from build123d import *

# Parameters (mm, degrees)
F0_R     = 39.5
F0_R_2   = 10.25
F1_DEPTH = 2
F2_R     = 11.25
F2_R_2   = 10.25
F3_DEPTH = 68
F4_R     = 12.5
F5_DEPTH = 1
F6_R     = 39.5
F6_R_2   = 10.25
F7_DEPTH = 2
F8_R     = 12.5
F9_DEPTH = 1


with BuildPart() as f1:
    # F0 (on Front) → F1 (new body)
    with BuildSketch(Plane.XZ):
        Circle(F0_R)
        Circle(F0_R_2, mode=Mode.SUBTRACT)
    extrude(amount=F1_DEPTH)

    # F2 (on face) → F3 (join)
    with BuildSketch(Plane.XZ.offset(2)):
        Circle(F2_R)
        Circle(F2_R_2, mode=Mode.SUBTRACT)
    extrude(amount=F3_DEPTH)

    # F4 (on face) → F5 (cut)
    with BuildSketch(Plane(origin=(0, 0, 0), x_dir=(-1, 0, 0), z_dir=(0, 1, 0))):
        Circle(F4_R)
    extrude(amount=-F5_DEPTH, mode=Mode.SUBTRACT)

    # F6 (on face) → F7 (join)
    with BuildSketch(Plane.XZ.offset(70)):
        Circle(F6_R)
        Circle(F6_R_2, mode=Mode.SUBTRACT)
    extrude(amount=F7_DEPTH)

    # F8 (on face) → F9 (cut)
    with BuildSketch(Plane.XZ.offset(72)):
        Circle(F8_R)
    extrude(amount=-F9_DEPTH, mode=Mode.SUBTRACT)


solid = f1.part
The listing builds one solid part. Answer for the finished solid, in the listing's coordinates (mm). A direction names the side the tool comes from. Give positions to 0.01 mm unless a question says otherwise; leave off trailing zeros. Write each loop counter-clockwise with the first axis right and the second up, starting at its lowest first coordinate (ties: lowest second). Pieces come first, ordered by that corner, then holes.
Item 1: Section D-D, the plane z = -26.5 is taken. Write down the section's boundary in (x, y), plus the area to 3 significant figures.
Item 2: Section C-C, the plane y = -51.5 is taken. Write down the section's boundary in (x, z).
Item 3: Flat-ended cylindrical pins translate along their axes: P1, Ø12, axis at x = 0.5, y = -28.5, coming from the +Z side; P2, Ø4, axis at x = -9.5, y = -30.5, coming from the -Z side; P3, Ø5, axis at y = -62, z = 1, coming from the -X side. Find the tip coordinate at first contact, or state that the pin passes through.
Item 4: Section A-A, the plane z = 0 is taken. Write down the section's boundary in (x, y), plus the area to 3 significant figures.
Item 5: Which of the six approach directions +Z, -Z, +X, -X, +Y, -Y give full straight-line access (tool end or side, diameter ignored) to faces 4 (the flat face through (1.91, -1, 10.24)), 5 (the flat face through (-1.91, -71, 10.24)), 6 (the flat face through (8.2, -2, -8.2))?
Item 6: Section B-B, the plane x = 0 is taken. Write down the section's boundary in (y, z), plus the area to 3 significant figures.
Item 7: Find the intervals of material crossed by line 1 along Y through (x, z) = (-15.5, -24); line 2 along Z through (x, y) = (0, -0.35); line 3 along Z through (x, y) = (0, -36), in increasing order.
Item 8: Determine the mould class of faces 1 (the flat face through (8.2, -70, -8.2)), 2 (the cylindrical face through (5.19, -35.52, -9.98)), 3 (the cylindrical face through (-11.923, -0.493, 3.755)) for opening direction Z: released by +Z, released by -Z, zero draft, split by the parting line, or undercut.
Completed:
1. outline: (-29.29, -72) - (29.29, -72) - (29.29, -70) - (-29.29, -70) - close; (-29.29, -2) - (29.29, -2) - (29.29, 0) - (-29.29, 0) - close
1. area: 234 mm2
2. outline: circle Ø22.5 at (0, 0); hole circle Ø20.5 at (0, 0)
3. P1: stops at z = 11.25
3. P2: stops at z = -8.39
3. P3: stops at x = -11.25
4. outline: (-39.5, -72) - (-12.5, -72) - (-12.5, -71) - (-10.25, -71) - (-10.25, -1) - (-12.5, -1) - (-12.5, 0) - (-39.5, 0) - (-39.5, -2) - (-11.25, -2) - (-11.25, -70) - (-39.5, -70) - close; (10.25, -71) - (12.5, -71) - (12.5, -72) - (39.5, -72) - (39.5, -70) - (11.25, -70) - (11.25, -2) - (39.5, -2) - (39.5, 0) - (12.5, 0) - (12.5, -1) - (10.25, -1) - close
4. area: 361 mm2
5. face 4: +Y
5. face 5: -Y
5. face 6: none
6. outline: (-72, -39.5) - (-70, -39.5) - (-70, -11.25) - (-2, -11.25) - (-2, -39.5) - (0, -39.5) - (0, -12.5) - (-1, -12.5) - (-1, -10.25) - (-71, -10.25) - (-71, -12.5) - (-72, -12.5) - close; (-72, 12.5) - (-71, 12.5) - (-71, 10.25) - (-1, 10.25) - (-1, 12.5) - (0, 12.5) - (0, 39.5) - (-2, 39.5) - (-2, 11.25) - (-70, 11.25) - (-70, 39.5) - (-72, 39.5) - close
6. area: 361 mm2
7. line 1: y = -72 to -70, -2 to 0
7. line 2: z = -39.5 to -12.5, 12.5 to 39.5
7. line 3: z = -11.25 to -10.25, 10.25 to 11.25
8. face 1: zero draft
8. face 2: split by the parting line
8. face 3: undercut
